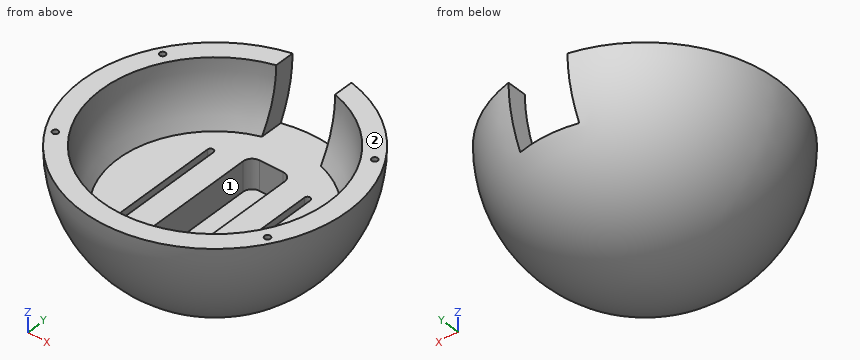
from build123d import *

# Parameters (mm, degrees)
F2_R     = 1.27
F3_DEPTH = 12.7
F5_DEPTH = 12.7
F6_W     = 25.4
F6_H     = 42.3964354956
F7_DEPTH = 25.4


with BuildPart() as f1:
    # F0 (on Front) → F1 (revolve)
    with BuildSketch(Plane.XZ):
        with BuildLine():
            Line((-48.895, 0), (-57.15, 0))
            ThreePointArc((-57.15, 0), (-40.4111525448, -40.4111525448), (0, -57.15))
            Line((0, -57.15), (0, -25.4))
            Line((0, -25.4), (-41.77991174, -25.4))
            ThreePointArc((-41.77991174, -25.4), (-47.0826391015, -13.188863493), (-48.895, 0))
        make_face()
    revolve(axis=Axis((0, 0, -41.275), (0, 0, -1)))

    # F2 (on face) → F3 (cut)
    with BuildSketch(Plane.XY):
        with Locations((45.72, 27.94)):
            Circle(F2_R)
        with Locations((45.72, -27.94)):
            Circle(F2_R)
        with Locations((-45.72, -27.94)):
            Circle(F2_R)
        with Locations((-45.72, 27.94)):
            Circle(F2_R)
    extrude(amount=-F3_DEPTH, mode=Mode.SUBTRACT)

    # F4 (on face) → F5 (cut)
    with BuildSketch(Plane.XY.offset(-25.4)):
        with BuildLine():
            Line((-20.88995587, -1.27), (-20.88995587, 0))
            Line((-20.88995587, 0), (-20.88995587, 1.27))
            ThreePointArc((-20.88995587, 1.27), (-21.7879814821, 0.8980256121), (-22.15995587, 0))
            ThreePointArc((-22.15995587, 0), (-21.7879814821, -0.8980256121), (-20.88995587, -1.27))
        make_face()
        with BuildLine():
            Line((-20.88995587, 1.27), (-20.88995587, 0))
            Line((-20.88995587, 0), (-20.88995587, -1.27))
            ThreePointArc((-20.88995587, -1.27), (-19.9919302579, -0.8980256121), (-19.61995587, 0))
            ThreePointArc((-19.61995587, 0), (-19.9919302579, 0.8980256121), (-20.88995587, 1.27))
        make_face()
        with BuildLine():
            ThreePointArc((-22.15995587, 0), (-21.7879814821, 0.8980256121), (-20.88995587, 1.27))
            ThreePointArc((-20.88995587, 1.27), (-19.9919302579, 0.8980256121), (-19.61995587, 0))
            Line((-19.61995587, 0), (-19.61995587, 22.86))
            ThreePointArc((-19.61995587, 22.86), (-20.88995587, 24.13), (-22.15995587, 22.86))
            Line((-22.15995587, 22.86), (-22.15995587, 0))
        make_face()
        with BuildLine():
            ThreePointArc((-19.61995587, 0), (-19.9919302579, -0.8980256121), (-20.88995587, -1.27))
            ThreePointArc((-20.88995587, -1.27), (-21.7879814821, -0.8980256121), (-22.15995587, 0))
            Line((-22.15995587, 0), (-22.15995587, -22.86))
            ThreePointArc((-22.15995587, -22.86), (-20.88995587, -24.13), (-19.61995587, -22.86))
            Line((-19.61995587, -22.86), (-19.61995587, 0))
        make_face()
        with BuildLine():
            Line((20.88995587, -1.27), (20.88995587, 0))
            Line((20.88995587, 0), (20.88995587, 1.27))
            ThreePointArc((20.88995587, 1.27), (19.9919302579, 0.8980256121), (19.61995587, 0))
            ThreePointArc((19.61995587, 0), (19.9919302579, -0.8980256121), (20.88995587, -1.27))
        make_face()
        with BuildLine():
            Line((20.88995587, 1.27), (20.88995587, 0))
            Line((20.88995587, 0), (20.88995587, -1.27))
            ThreePointArc((20.88995587, -1.27), (21.7879814821, -0.8980256121), (22.15995587, 0))
            ThreePointArc((22.15995587, 0), (21.7879814821, 0.8980256121), (20.88995587, 1.27))
        make_face()
        with BuildLine():
            ThreePointArc((19.61995587, 0), (19.9919302579, 0.8980256121), (20.88995587, 1.27))
            ThreePointArc((20.88995587, 1.27), (21.7879814821, 0.8980256121), (22.15995587, 0))
            Line((22.15995587, 0), (22.15995587, 22.86))
            ThreePointArc((22.15995587, 22.86), (20.88995587, 24.13), (19.61995587, 22.86))
            Line((19.61995587, 22.86), (19.61995587, 0))
        make_face()
        with BuildLine():
            ThreePointArc((22.15995587, 0), (21.7879814821, -0.8980256121), (20.88995587, -1.27))
            ThreePointArc((20.88995587, -1.27), (19.9919302579, -0.8980256121), (19.61995587, 0))
            Line((19.61995587, 0), (19.61995587, -22.86))
            ThreePointArc((19.61995587, -22.86), (20.88995587, -24.13), (22.15995587, -22.86))
            Line((22.15995587, -22.86), (22.15995587, 0))
        make_face()
        with BuildLine():
            Line((5.08, 29.21), (-5.08, 29.21))
            ThreePointArc((-5.08, 29.21), (-7.7740768363, 28.0940768363), (-8.89, 25.4))
            Line((-8.89, 25.4), (-8.89, -25.4))
            ThreePointArc((-8.89, -25.4), (-7.7740768363, -28.0940768363), (-5.08, -29.21))
            Line((-5.08, -29.21), (5.08, -29.21))
            ThreePointArc((5.08, -29.21), (7.7740768363, -28.0940768363), (8.89, -25.4))
            Line((8.89, -25.4), (8.89, 25.4))
            ThreePointArc((8.89, 25.4), (7.7740768363, 28.0940768363), (5.08, 29.21))
        make_face()
    extrude(amount=-F5_DEPTH, mode=Mode.SUBTRACT)

    # F6 (on face) → F7 (cut)
    with BuildSketch(Plane.XY):
        with Locations((0, 51.4418943548)):
            Rectangle(F6_W, F6_H)
    extrude(amount=-F7_DEPTH, mode=Mode.SUBTRACT)


solid = f1.part
CAD build for the part. Positions are in the model's coordinates, mm. Face numbers are marked on the shaded views. Give positions to 0.01 mm unless a question says otherwise; leave off trailing zeros. Loops run counter-clockwise (first coordinate to the right, second up) from the corner with the lowest first, then second, coordinate; pieces in that order, holes last. Notation, with made-up numbers: M 1,-13.75 L 49,-13.75 A22 ccw 49,-3.75 Z; hole C 64.25,-19 d3. An arc over 180 degrees is marked long. Answer in a Markdown table with one row per item. Add a question column.
Item 1: Band-saw the part on A-A on y = 43.5. Give the cut face in (x, z), then the cut area to 3 significant figures.
Item 2: Band-saw the part on B-B on z = -47. Give the cut face in (x, y), then the cut area to 3 significant figures.
Item 3: Band-saw the part on C-C on x = -27.5. Give the cut face in (y, z), then the cut area to 3 significant figures.
Item 4: Drop flat-ended pins along their axis: P1, Ø14, axis at y = 11, z = -29, coming from the -X side; P2, Ø4, axis at x = -25, z = -28, coming from the -Y side; P3, Ø4, axis at y = -7, z = -28.5, coming from the -X side. Give the stop position or say it passes through.
Item 5: Band-saw the part on D-D on z = -17.5. Give the cut face in (x, y).
Item 6: Probe probe 1 along Y at (x, z) = (45, -6); probe 2 along Y at (x, z) = (45, -5); probe 3 along X at (y, z) = (27, -6). List the from-to ranges inside material, lowest first.
Item 7: Mould opens along X. For the marked faces 1 and 2 say: +X half, -X half, draft (parallel to the pull), parting line (faces both ways), or undercut.
Reply:
| question | item | result |
|---|---|---|
| 1 | outline | M -37.07,0 A37.07 ccw 37.07,0 L 22.33,0 A22.33 cw 12.7,-18.36 L 12.7,-25.4 L -12.7,-25.4 L -12.7,-18.36 A22.33 cw -22.33,0 Z |
| 1 | area | 1,260 mm^2 |
| 2 | outline | C 0,0 d65.03 |
| 2 | area | 3,320 mm^2 |
| 3 | outline | M -50.1,0 A50.1 ccw 50.1,0 L 40.43,0 A40.43 cw 31.45,-25.4 L -31.45,-25.4 A40.43 cw -40.43,0 Z |
| 3 | area | 2,030 mm^2 |
| 4 | P1 | stops at x = -51.86 |
| 4 | P2 | stops at y = -44.76 |
| 4 | P3 | stops at x = -50.18 |
| 5 | outline | M -12.7,43.85 L -12.7,52.9 A54.4 ccw long 12.7,52.9 L 12.7,43.85 A45.66 cw long Z |
| 6 | probe 1 | y = -34.71 to -28.99, -26.89 to -18.16, 18.16 to 26.89, 28.99 to 34.71 |
| 6 | probe 2 | y = -34.87 to -28.99, -26.89 to -18.46, 18.46 to 26.89, 28.99 to 34.87 |
| 6 | probe 3 | x = -50.01 to -46.57, -44.87 to -40.32, 40.32 to 44.87, 46.57 to 50.01 |
| 7 | face 1 | undercut |
| 7 | face 2 | draft |
